Verification items for this drawing (mm, ordinates from the low corner). Coordinates: 2 decimals unless noted, no trailing zeros. Loops run counter-clockwise (first coordinate to the right, second up) from the corner with the lowest first, then second, coordinate; pieces in that order, holes last. Notation, with made-up numbers: M -33.75,-38 L -11.75,-38 A28 cw -11.75,-7 Z; hole C 86,49.5 d7. An arc over 180 degrees is marked long. Return JSON: item names as keys, results as strings.
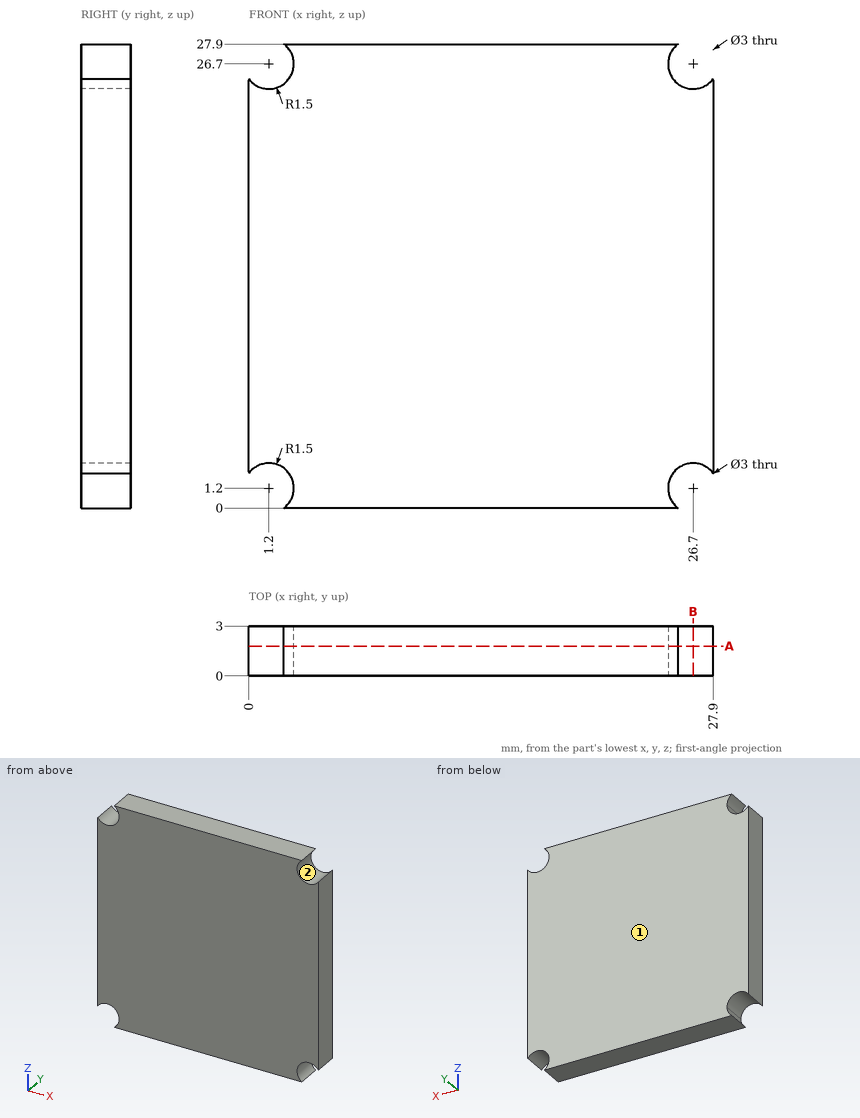
1) Go/stop test with a flat-tipped pin: pin 1 Ø1.8 at (x, z) = (26.7, 1.2) entering from +Y. Record where the tip stops, or that it passes through.
Answers:
{"pin 1": "through"}
2) Draft check along X on the marked faces 1 and 2. Enter one of: +X half, -X half, draft (parallel to the pull), parting line (faces both ways), or undercut.
Answers:
{"face 1": "draft", "face 2": "undercut"}
3) Section check B-B on x = 26.7. Record the cut outline in (y, z), then the cut area to 3 significant figures.
Answers:
{"outline": "M 0,2.7 L 3,2.7 L 3,25.2 L 0,25.2 Z", "area": "67.5 mm²"}
4) Scan lines: line 1 along Z through (x, y) = (26.7, 1.5); line 2 along Z through (x, y) = (1.75, 2.5). Record each from-to range of solid material in increasing order. Write a range as [from, to].
Answers:
{"line 1": "[2.7, 25.2]", "line 2": "[2.6, 25.3]"}
5) Section check A-A on y = 1.8. Record the cut outline in (x, z).
Answers:
{"outline": "M 0,2.1 A1.5 cw long 2.1,0 L 25.8,0 A1.5 cw long 27.9,2.1 L 27.9,25.8 A1.5 cw long 25.8,27.9 L 2.1,27.9 A1.5 cw long 0,25.8 Z"}
